For this review, take the finished solid that the model builds, in its own axes (mm). Round coordinates to 2 decimals unless told otherwise and drop trailing zeros. Order: outer loops, then holes, each group sorted by start corner. A loop starts at its lowest first (then second) coordinate and runs counter-clockwise, first axis right, second up. Notation, with made-up numbers: M 56,9 L 74,9 A30 ccw 74,35 Z; hole C -12,41 d3. An arc over 180 degrees is marked long. Answer in a Markdown table with one row per item. Add a question column.
Autodesk Inventor part; units mm, degrees
ref_plane "YZ Plane" through (0, 0, 0) normal (1, 0, 0) x (0, 1, 0)
ref_plane "XZ Plane" through (0, 0, 0) normal (0, 1, 0) x (-1, 0, 0)
ref_plane "XY Plane" through (0, 0, 0) normal (0, 0, 1) x (1, 0, 0)
sketch "Sketch1" plane through (0, 0, 0) normal (1, 0, 0) x (0, 1, 0)
  line L0 (48.3789, 0) -> (148.3789, 0)
  line L1 (248.3789, -333.1357) -> (248.3789, -336.1798)
  line L2 (148.3789, -400) -> (48.3789, -400)
  line L3 (48.3789, -400) -> (48.3789, 0)
  line L4 (198.3789, -260) -> (48.3789, -260)
  line L5 (48.3789, -260) -> (48.3789, -140)
  line L6 (48.3789, -140) -> (198.3789, -140)
  line L7 (198.3789, -140) -> (198.3789, -260)
  line L8 (-98.7773, -200) -> (409.3156, -200)
  arc A0 (298.3789, -200) -> (148.3789, 0) centre (92.075, -198.478) ccw
  arc A1 (148.3789, -400) -> (298.3789, -200) centre (92.075, -201.522) ccw
  point P0 (248.3789, -63.8202)
  point P1 (248.3789, -200)
  dimension "d11" = 120
  dimension "d12" = 150
  dimension "d13" = 50
  dimension "d14" = 140
  dimension "d18" = 200
  dimension "d19" = 200
  dimension "d20" = 50
  dimension "d21" = 100
  dimension "d23" = 400
extrude "Extrusion1" add sketch "Sketch1" along normal blind 10 contours L0 A0 L8 L7 L6 L3 | A1 L2 L3 L4 L7 L8
properties part number "beam"
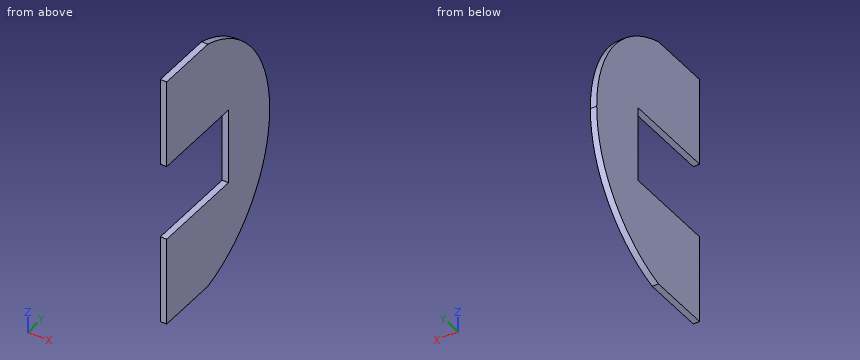
1. Consider section D-D on y = 232.5. Write out the cut boundary in (x, z).
2. To check wall thickness, follow probe 1 along Z at (x, y) = (2.25, 89); probe 2 along Y at (x, z) = (8.25, -200.5); probe 3 along Z at (x, y) = (5.5, 202.5). State the ranges of each line that lie inside material, in increasing order. Write a range as [from, to].
3. Consider section C-C on z = -56. Write out the cut boundary in (x, y), plus the area to 3 significant figures.
4. Consider section A-A on y = 84. Write out the cut boundary in (x, z).
5. Clearance check with flat-ended pins moving along their axes: pin 1 Ø5 at (x, z) = (7, -210) entering from -Y; pin 2 Ø4 at (x, z) = (3.5, -208) entering from +Y; pin 3 Ø2 at (x, z) = (9, -274) entering from +Y. State where each tip first meets the part, or that it passes through.
6. Consider section B-B on x = 2. Write out the cut boundary in (y, z).
Solved:
| question | item | result |
|---|---|---|
| 1 | outline | M 0,-352.67 L 10,-352.67 L 10,-47.33 L 0,-47.33 Z |
| 2 | probe 1 | z = [-400, -260], [-140, 0] |
| 2 | probe 2 | y = [198.38, 298.38] |
| 2 | probe 3 | z = [-375.79, -24.21] |
| 3 | outline | M 0,48.38 L 10,48.38 L 10,241.29 L 0,241.29 Z |
| 3 | area | 1,930 mm^2 |
| 4 | outline | M 0,-400 L 10,-400 L 10,-260 L 0,-260 Z; M 0,-140 L 10,-140 L 10,0 L 0,0 Z |
| 5 | pin 1 | stops at y = 198.38 |
| 5 | pin 2 | stops at y = 298.34 |
| 5 | pin 3 | stops at y = 285.61 |
| 6 | outline | M 48.38,-400 L 148.38,-400 A206.31 ccw 298.38,-200 A206.31 ccw 148.38,0 L 48.38,0 L 48.38,-140 L 198.38,-140 L 198.38,-260 L 48.38,-260 Z |
